Source: CAD feature listing. Evaluate the final solid. Frame: model axes, mm. Face numbers are marked on the shaded views. A direction names the side the tool comes from. Give positions to 0.01 mm unless a question says otherwise; leave off trailing zeros. Loops run counter-clockwise (first coordinate to the right, second up) from the corner with the lowest first, then second, coordinate; pieces in that order, holes last. Notation, with made-up numbers: (58, 80.5) -> (109, 80.5) arc R15 ccw to (109, 89.5) -> close; hole circle Ø4 at (-28.75, -16). An arc over 180 degrees is marked (long way). Return JSON: item names as keys, results as strings. Group by question number.
(1) Draft query along X for the marked faces 1, 2 and 3. Return one class per face: released by +X, released by -X, zero draft, split by the parting line, or undercut.
(2) Pin query (flat end, axial travel): pin 1 (3 mm diameter, centred on x = 0, z = 7, fed in from -Y); pin 2 (0.8 mm diameter, centred on x = 0, z = 3.5, fed in from +Y). Return the tip coordinate at first contact, or that it passes through.
(3) Cut plane A-A on y = 0.75. Return loops of the section in (x, z) (3 decimals), then the cut area to 3 significant figures.
(4) Access query for the marked faces 4 and 5. Directions: +Z, -Z, +X, -X, +Y, -Y. A direction counts if a zero-diameter tool reaches every point of the face in a straight line with its end or side. Return the directions, or none.
(5) Ray query, line 1 (X direction, y = 0.5, z = 0) (3 decimals); line 2 (Y direction, x = 6.75, z = 3.25); line 3 (Z direction, x = -1.5, y = -0.9). Return the intervals inside material, ascending. Write a range as from..to.
```python
from build123d import *

# Parameters (mm, degrees)
SKETCH1_R           = 10
BOSS_EXTRUDE1_DEPTH = 2
SKETCH2_R           = 4.5
BOSS_EXTRUDE2_DEPTH = 2.5
SKETCH3_R           = 1.275
CUT_EXTRUDE1_DEPTH  = 15.361406616
FILLET1_R           = 0.25
SKETCH6_R           = 1
CUT_EXTRUDE2_DEPTH  = 15.840822214
SKETCH7_R           = 2.9
CUT_EXTRUDE3_DEPTH  = 2.5
BOSS_EXTRUDE4_DEPTH = 2.5
CIRPATTERN1_COUNT   = 26
SKETCH9_W           = 1
SKETCH9_H           = 7
CUT_EXTRUDE4_DEPTH  = 0.5


with BuildPart() as part:
    # Sketch1 → Boss-Extrude1 (new body)
    with BuildSketch(Plane(origin=(0, 0, 0), x_dir=(1, 0, 0), z_dir=(0, 1, 0))):
        with Locations(Location((0, 0, 0), (0, 0, 270))):
            Circle(SKETCH1_R)
    extrude(amount=BOSS_EXTRUDE1_DEPTH)

    # Sketch2 → Boss-Extrude2 (add)
    with BuildSketch(Plane(origin=(0, 0, 0), x_dir=(1, 0, 0), z_dir=(0, 1, 0))):
        with Locations(Location((0, 0, 0), (0, 0, 270))):
            Circle(SKETCH2_R)
    extrude(amount=-BOSS_EXTRUDE2_DEPTH)

    # Sketch3 → Cut-Extrude1 (cut, through all)
    with BuildSketch(Plane(origin=(0, 0, 0), x_dir=(1, 0, 0), z_dir=(0, 1, 0))):
        with Locations(Location((0, 7, 0), (0, 0, 270))):
            Circle(SKETCH3_R)
        with Locations(Location((-7, 0, 0), (0, 0, 270))):
            Circle(SKETCH3_R)
        with Locations(Location((0, -7, 0), (0, 0, 90))):
            Circle(SKETCH3_R)
        with Locations(Location((7, 0, 0), (0, 0, 90))):
            Circle(SKETCH3_R)
    extrude(amount=CUT_EXTRUDE1_DEPTH, mode=Mode.SUBTRACT)

    # Fillet1
    fillet1_edges = [part.edges().sort_by_distance(p)[0] for p in [
        (0, 0, -10),
    ]]
    fillet(fillet1_edges, radius=FILLET1_R)

    # Sketch6 → Cut-Extrude2 (cut, through all)
    with BuildSketch(Plane(origin=(0, 2, 0), x_dir=(1, 0, 0), z_dir=(0, 1, 0))):
        with Locations(Location((0, 0, 0), (0, 0, 270))):
            Circle(SKETCH6_R)
    extrude(amount=-CUT_EXTRUDE2_DEPTH, mode=Mode.SUBTRACT)

    # Sketch7 → Cut-Extrude3 (cut)
    with BuildSketch(Plane.XZ.offset(2.5)):
        with Locations(Location((0, 0, 0), (0, 0, 270))):
            Circle(SKETCH7_R)
    extrude(amount=-CUT_EXTRUDE3_DEPTH, mode=Mode.SUBTRACT)

    # Sketch8 → Boss-Extrude4 (add)
    with BuildSketch(Plane.XZ.offset(2.5)):
        with BuildLine():
            Line((-2.35244742, -1.046531787), (-2.745588284, -0.933672842))
            ThreePointArc((-2.745588284, -0.933672842), (-2.649635472, -1.178741646), (-2.531859978, -1.414102207))
            Line((-2.531859978, -1.414102207), (-2.35244742, -1.046531787))
        make_face()
    boss_extrude4 = extrude(amount=-BOSS_EXTRUDE4_DEPTH)

    # CirPattern1: Boss-Extrude4 ×26 about axis
    cirpattern1_axis = Axis((0, 0, 0), (0, 1, 0))
    for i in range(1, CIRPATTERN1_COUNT):
        add(boss_extrude4.rotate(cirpattern1_axis, i * 360 / CIRPATTERN1_COUNT))

    # Sketch9 → Cut-Extrude4 (cut)
    with BuildSketch(Plane(origin=(0, 2, 0), x_dir=(1, 0, 0), z_dir=(0, 1, 0))):
        with Locations((0, -3.5)):
            Rectangle(SKETCH9_W, SKETCH9_H)
    extrude(amount=-CUT_EXTRUDE4_DEPTH, mode=Mode.SUBTRACT)


solid = part.part
```
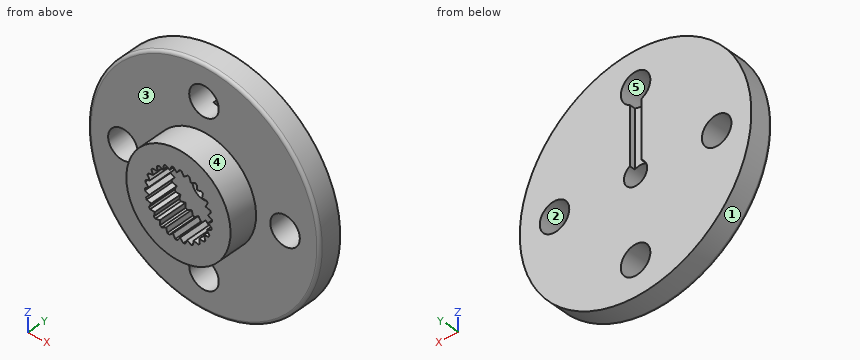
Answers:
{
 "1": {"face 1": "split by the parting line", "face 2": "undercut", "face 3": "zero draft"},
 "2": {"pin 1": "y = 0", "pin 2": "y = 1.5"},
 "3": {"outline": "circle Ø20 at (0, 0); hole circle Ø2.55 at (-7, 0); hole circle Ø2.55 at (0, -7); hole circle Ø2.55 at (0, 7); hole circle Ø2 at (0, 0); hole circle Ø2.55 at (7, 0)", "area": "291 mm²"},
 "4": {"face 4": "-Y", "face 5": "+Y, -Y"},
 "5": {"line 1": "-10..-8.275, -5.725..-1, 1..5.725, 8.275..10", "line 2": "0..2", "line 3": "-4.24..-2.48, 2.27..4.24"}
}
